from build123d import *

# Parameters (mm, degrees)
F0_R     = 11.25
F1_DEPTH = 2
F2_R     = 6
F3_DEPTH = 1
F6_DEPTH = 6.5
F7_DEPTH = 6


with BuildPart() as f1:
    # F0 (on Top) → F1 (new body)
    with BuildSketch(Plane.XY):
        Circle(F0_R)
    extrude(amount=F1_DEPTH)

    # F2 (on face) → F3 (join)
    with BuildSketch(Plane.XY.offset(2)):
        Circle(F2_R)
    extrude(amount=F3_DEPTH)

    # F5 (on face) → F6 (join)
    with BuildSketch(Plane.XY.offset(3)):
        with BuildLine():
            ThreePointArc((0, 3.716564), (-3.978639, -0.033436), (0, -3.783436))
            Line((0, -3.783436), (0, 3.716564))
        make_face()
    extrude(amount=F6_DEPTH)

    # F5 (on face) → F7 (join)
    with BuildSketch(Plane.XY.offset(3)):
        with BuildLine():
            ThreePointArc((0, 3.716564), (-3.978639, -0.033436), (0, -3.783436))
            Line((0, -3.783436), (0, 3.716564))
        make_face()
    extrude(amount=F7_DEPTH)


solid = f1.part
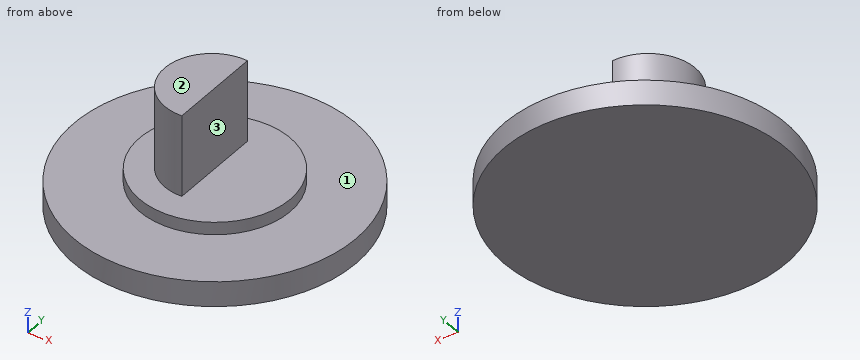
Build history of the part. All positions in model axes, mm. Face numbers are marked on the shaded views. A direction names the side the tool comes from. Coordinates: 2 decimals unless noted, no trailing zeros. Write each loop counter-clockwise with the first axis right and the second up, starting at its lowest first coordinate (ties: lowest second). Pieces come first, ordered by that corner, then holes.
(1) Pin check, flat tips, straight feed: pin 1 Ø1 at (x, z) = (-2, 4) entering from -Y; pin 2 Ø1.5 at (y, z) = (-8, 4.5) entering from -X; pin 3 Ø12 at (x, y) = (-7, -8.5) entering from +Z; pin 4 Ø4 at (y, z) = (-3.5, 1.5) entering from -X. Stop position of each tip, or through.
(2) Cut at D-D on x = -6.75. List the corners of the cut face in (y, z).
(3) 3-axis set-ups, long thin cutter, end or side, ignore diameter. For the marked faces 1, 2 and 3: which of +Z, -Z, +X, -X, +Y, -Y reach the whole face in a straight line?
(4) Cut at B-B on x = -4.5. List the corners of the cut face in (y, z), and give its area (3 significant figures).
(5) Cut at A-A on z = 1.5. List the corners of the cut face in (x, y), and give its area (3 significant figures).
(6) Cut at C-C on y = 4.25. List the corners of the cut face in (x, z), and give its area (3 significant figures).
(7) Drill centre lines: line 1 (Z direction, x = 3.25, y = 4.5); line 2 (Z direction, x = -8.5, y = 3.75); line 3 (Y direction, x = -2.5, z = 9.25). Where is each one in solid material? Low to high.
Working result:
1. pin 1: stops at y = -3.57
1. pin 2: passes through
1. pin 3: stops at z = 3
1. pin 4: stops at x = -11.15
2. outline: (-9, 0) - (9, 0) - (9, 2) - (-9, 2) - close
3. face 1: +Z
3. face 2: +Z, +X, -X, +Y, -Y
3. face 3: +Z, +X, +Y, -Y
4. outline: (-10.31, 0) - (10.31, 0) - (10.31, 2) - (3.97, 2) - (3.97, 3) - (-3.97, 3) - (-3.97, 2) - (-10.31, 2) - close
4. area: 49.2 mm2
5. outline: circle Ø22.5 at (0, 0)
5. area: 398 mm2
6. outline: (-10.42, 0) - (10.42, 0) - (10.42, 2) - (4.24, 2) - (4.24, 3) - (-4.24, 3) - (-4.24, 2) - (-10.42, 2) - close
6. area: 50.1 mm2
7. line 1: z = 0 to 3
7. line 2: z = 0 to 2
7. line 3: y = -3.02 to 2.95
